Could you check a few things on this model? Use its own coordinates, in mm. A direction names the side the tool comes from. Coordinates: 2 decimals unless noted, no trailing zeros. Order: outer loops, then holes, each group sorted by start corner. A loop starts at its lowest first (then second) coordinate and runs counter-clockwise, first axis right, second up. Notation, with made-up numbers: (-17, 4.25) -> (37, 4.25) arc R12 cw to (37, 9.25) -> close; hole circle Ø11 at (37.5, 84.5). An arc over 180 degrees is marked (long way). Put each result on its own line as item: value. Start each with the question number.
Q1. For faces 1 (the face through (1, 0, 0)), 2 (the face through (-0.508, -4, 1)), which set-ups out of +Z, -Z, +X, -X, +Y, -Y let a thin tool reach every point of the face, with its end or its side?
Q2. If we section it at C-C (z = 0.2): Please give me the cut outline in (x, y) (1 decimal).
Q3. If we section it at D-D (x = 3): Please give me the cut outline in (y, z).
Q4. If we section it at A-A (x = 0): Please give me the cut outline in (y, z) (3 decimals).
Q5. Will this pin go through, and if not, where does the flat tip stop? pin 1 (0.8 mm diameter, centred on x = 0, y = 0, fed in from +Z).
Q6. If we section it at B-B (y = -0.5): Please give me the cut outline in (x, z), and give its area (3 significant figures).
Q7. We'd pull the mould along Y, two halves only. Please class faces 3 (the face through (-0.08, 0.63, 0.63)), 4 (the face through (0.508, -4, 1)), 5 (the face through (0, -4.645, 1)): +Y half, -Y half, draft (parallel to the pull), parting line (faces both ways), or undercut.
Q8. Please list where these lines run through material, in increasing order: line 1 along Y through (x, z) = (0, 0.55) (3 decimals); line 2 along X through (y, z) = (0.5, 0.4); line 3 along Y through (x, z) = (0.25, 1.15).
from build123d import *

# Parameters (mm, degrees)
F0_R     = 0.635
F0_R_2   = 0.1905
F1_DEPTH = 1.27


with BuildPart() as f1:
    # F0 (on Top) → F1 (new body)
    with BuildSketch(Plane.XY):
        with BuildLine():
            ThreePointArc((0.508, -3.7759814618), (2.8680638068, -2.5080490426), (3.81, 0))
            ThreePointArc((3.81, 0), (-2.5080490426, 2.8680638068), (-0.508, -3.7759814618))
            Line((-0.508, -3.7759814618), (-0.508, -2.1051138332))
            Line((-0.508, -2.1051138332), (0.508, -2.1051138332))
            Line((0.508, -2.1051138332), (0.508, -3.7759814618))
        make_face()
        Circle(F0_R, mode=Mode.SUBTRACT)
        with Locations((0, 3.1728937756)):
            Circle(F0_R_2, mode=Mode.SUBTRACT)
        with BuildLine():
            Line((-0.508, -2.1051138332), (-0.508, -3.7759814618))
            ThreePointArc((-0.508, -3.7759814618), (0, -3.81), (0.508, -3.7759814618))
            Line((0.508, -3.7759814618), (0.508, -2.1051138332))
            Line((0.508, -2.1051138332), (-0.508, -2.1051138332))
        make_face()
        with BuildLine():
            ThreePointArc((0.508, -3.7759814618), (0, -3.81), (-0.508, -3.7759814618))
            Line((-0.508, -3.7759814618), (-0.508, -4.6451138332))
            Line((-0.508, -4.6451138332), (0.508, -4.6451138332))
            Line((0.508, -4.6451138332), (0.508, -3.7759814618))
        make_face()
    extrude(amount=F1_DEPTH)


solid = f1.part
The answers:
1. face 1: -Z, +X, -X, +Y, -Y
1. face 2: +Z, -Z, -X, -Y
2. outline: (-0.5, -4.6) -> (0.5, -4.6) -> (0.5, -3.8) arc R3.8 ccw (long way) to (-0.5, -3.8) -> close; hole circle Ø1.3 at (0, 0); hole circle Ø0.4 at (0, 3.2)
3. outline: (-2.35, 0) -> (2.35, 0) -> (2.35, 1.27) -> (-2.35, 1.27) -> close
4. outline: (-4.645, 0) -> (-0.635, 0) -> (-0.635, 1.27) -> (-4.645, 1.27) -> close; (0.635, 0) -> (2.982, 0) -> (2.982, 1.27) -> (0.635, 1.27) -> close; (3.363, 0) -> (3.81, 0) -> (3.81, 1.27) -> (3.363, 1.27) -> close
5. pin 1: through
6. outline: (-3.78, 0) -> (-0.39, 0) -> (-0.39, 1.27) -> (-3.78, 1.27) -> close; (0.39, 0) -> (3.78, 0) -> (3.78, 1.27) -> (0.39, 1.27) -> close
6. area: 8.60 mm^2
7. face 3: undercut
7. face 4: draft
7. face 5: -Y half
8. line 1: -4.645 to -0.635, 0.635 to 2.982, 3.363 to 3.81
8. line 2: -3.78 to -0.39, 0.39 to 3.78
8. line 3: -4.65 to -0.58, 0.58 to 3.8
